Input: part model. Units: mm. Frame: model coordinates. Coordinates: 2 decimals unless noted, no trailing zeros. Write each loop counter-clockwise with the first axis right and the second up, starting at its lowest first coordinate (ties: lowest second). Pieces come first, ordered by that corner, then holes. Notation, with made-up numbers: (6.5, -19.5) -> (49.5, -19.5) arc R10 ccw to (49.5, -8.5) -> close; hole circle Ø4 at (40.5, -38.5). An arc over 180 degrees is marked (long way). One line per question, with ' | ' between items. Start each with the question number.
Autodesk Inventor part; units mm, degrees
ref_plane "Plan YZ" through (0, 0, 0) normal (1, 0, 0) x (0, 1, 0)
ref_plane "Plan XZ" through (0, 0, 0) normal (0, 1, 0) x (-1, 0, 0)
ref_plane "Plan XY" through (0, 0, 0) normal (0, 0, 1) x (1, 0, 0)
sketch "Esquisse1" plane through (0, 0, 0) normal (0, 0, 1) x (1, 0, 0)
  line L0 (4, 3) -> (36, 3)
  line L1 (36, 103) -> (4, 103)
  line L2 (0, 106) -> (4, 106)
  line L3 (4, 106) -> (4, 103)
  line L4 (40, 106) -> (36, 106)
  line L5 (36, 106) -> (36, 103)
  line L6 (0, 0) -> (4, 0)
  line L7 (4, 0) -> (4, 3)
  line L8 (36, 3) -> (36, 0)
  line L9 (36, 0) -> (40, 0)
  line L10 (40, 0) -> (40, 106)
  line L11 (0, 0) -> (0, 106)
  dimension "d6" = 100
  dimension "d8" = 3
  dimension "d9" = 3
  dimension "d13" = 40
  dimension "d14" = 4
  dimension "d15" = 4
extrude "Extrusion1" add sketch "Esquisse1" along normal blind 3
sketch "Esquisse6" plane through (0, 0, 3) normal (0, 0, 1) x (1, 0, 0)
  line L0 (0, 106) -> (0, 0)
  line L1 (40, 0) -> (40, 106)
  line L2 (0, -646.5316) -> (20, -646.5316) construction
  line L3 (40, -683.5995) -> (20, -683.5995) construction
  line L4 (20, 88.2545) -> (20, 14.0947) construction
  circle A0 centre (20, 83) radius 3.9
  circle A1 centre (20, 63) radius 3.9
  line L5 (36, 103) -> (4, 103)
  line L6 (36, 0) -> (40, 0)
  dimension "d18" = 20
  dimension "d19" = 20
  dimension "d20" = 7.8
  dimension "d21" = 7.8
extrude "Extrusion2" cut sketch "Esquisse6" against normal through all
sketch "Esquisse7" plane through (0, 0, 3) normal (0, 0, 1) x (1, 0, 0)
  line L0 (40, 0) -> (40, 106) construction
  line L1 (0, 106) -> (0, 0) construction
  line L2 (20, 50.9423) -> (20, 15.6231) construction
  line L3 (0, 42.5223) -> (20, 42.5223) construction
  line L4 (20, 46.099) -> (40, 46.099) construction
  line L5 (36, 0) -> (40, 0)
  point P0 (20, 30)
  dimension "d27" = 30
hole "Perçage1" at (20, 30, 3) direction (0, 0, -1) diameter 2.459 end through all
properties part number "S1702_paroiinterne" material "Plastique PMMA"
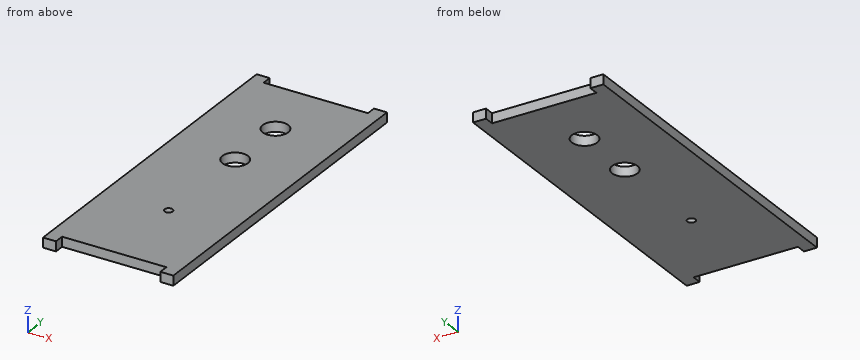
1) Section C-C, the plane z = 2.1. Return loops of the section in (x, y).
2) Section A-A, the plane x = 20. Return loops of the section in (y, z).
3) First-contact query: P1, Ø0.9, axis at x = 22.5, z = 2, coming from the -Y side. Flat tip, straight axial feed; report the tip coordinate or a pass-through.
4) Section D-D, the plane y = 30. Return loops of the section in (x, z).
5) Section B-B, the plane y = 63. Return loops of the section in (x, z), then the cut area to 3 significant figures.
6) Ray query, line 1 (Y direction, x = 20, z = 1.35); line 2 (Y direction, x = 21, z = 1.6); line 3 (Y direction, x = 23.5, z = 2.6). Return the intervals inside material, ascending.
Answer block:
1) outline: (0, 0) -> (4, 0) -> (4, 3) -> (36, 3) -> (36, 0) -> (40, 0) -> (40, 106) -> (36, 106) -> (36, 103) -> (4, 103) -> (4, 106) -> (0, 106) -> close; hole circle Ø7.8 at (20, 63); hole circle Ø7.8 at (20, 83); hole circle Ø2.46 at (20, 30)
2) outline: (3, 0) -> (28.77, 0) -> (28.77, 3) -> (3, 3) -> close; (31.23, 0) -> (59.1, 0) -> (59.1, 3) -> (31.23, 3) -> close; (66.9, 0) -> (79.1, 0) -> (79.1, 3) -> (66.9, 3) -> close; (86.9, 0) -> (103, 0) -> (103, 3) -> (86.9, 3) -> close
3) P1: stops at y = 3
4) outline: (0, 0) -> (18.77, 0) -> (18.77, 3) -> (0, 3) -> close; (21.23, 0) -> (40, 0) -> (40, 3) -> (21.23, 3) -> close
5) outline: (0, 0) -> (16.1, 0) -> (16.1, 3) -> (0, 3) -> close; (23.9, 0) -> (40, 0) -> (40, 3) -> (23.9, 3) -> close | area: 96.6 mm2
6) line 1: y = 3 to 28.77, 31.23 to 59.1, 66.9 to 79.1, 86.9 to 103 | line 2: y = 3 to 29.28, 30.72 to 59.23, 66.77 to 79.23, 86.77 to 103 | line 3: y = 3 to 61.28, 64.72 to 81.28, 84.72 to 103
